from build123d import *

# Parameters (mm, degrees)
SKETCH_W        = 34
SKETCH_H        = 34
PAD_DEPTH       = 80
POCKET_DEPTH    = 80
SKETCH002_R     = 3
POCKET001_DEPTH = 4
SKETCH003_R     = 3
POCKET002_DEPTH = 4
SKETCH004_R     = 4
POCKET003_DEPTH = 2
SKETCH005_R     = 4
POCKET004_DEPTH = 2
SKETCH006_W     = 6.4
SKETCH006_H     = 2
SKETCH006_W_2   = 4
POCKET005_DEPTH = 12
SKETCH007_W     = 6.4
SKETCH007_H     = 2
SKETCH007_W_2   = 4
POCKET006_DEPTH = 12
CHAMFER_SIZE    = 1.98
CHAMFER001_SIZE = 1.98


with BuildPart() as part:
    # Sketch → Pad (new body)
    with BuildSketch(Plane.XY):
        with Locations((17, 17)):
            Rectangle(SKETCH_W, SKETCH_H)
    extrude(amount=PAD_DEPTH)

    # Sketch001 (on Face6 of Pad) → Pocket (cut)
    with BuildSketch(Plane.XY.offset(80)):
        Polygon((6.5, 27.5), (14, 27.5), (14, 23.5), (17, 21), (20, 23.5), (20, 27.5), (27.5, 27.5), (27.5, 19.5), (23.5, 19.5), (21, 17), (23.5, 14), (27.5, 14), (27.5, 6.5), (20, 6.5), (20, 10.5), (17, 13), (14, 10.5), (14, 6.5), (6.5, 6.5), (6.5, 14), (10.5, 14), (13, 17), (10.5, 19.5), (6.5, 19.5), align=None)
    extrude(amount=-POCKET_DEPTH, mode=Mode.SUBTRACT)

    # Sketch002 (on Face2 of Pocket) → Pocket001 (cut)
    with BuildSketch(Plane(origin=(0, 0, 0), x_dir=(0, -1, 0), z_dir=(-1, 0, 0))):
        with Locations((-17, 60)):
            Circle(SKETCH002_R)
        with Locations((-17, 20)):
            Circle(SKETCH002_R)
    extrude(amount=-POCKET001_DEPTH, mode=Mode.SUBTRACT)

    # Sketch003 (on Face3 of Pocket001) → Pocket002 (cut)
    with BuildSketch(Plane.YZ.offset(34)):
        with Locations((17, 60)):
            Circle(SKETCH003_R)
        with Locations((17, 20)):
            Circle(SKETCH003_R)
    extrude(amount=-POCKET002_DEPTH, mode=Mode.SUBTRACT)

    # Sketch004 (on Face1 of Pocket002) → Pocket003 (cut)
    with BuildSketch(Plane(origin=(0, 34, 0), x_dir=(-1, 0, 0), z_dir=(0, 1, 0))):
        with Locations((-27, 60)):
            Circle(SKETCH004_R)
        with Locations((-7, 60)):
            Circle(SKETCH004_R)
        with Locations((-27, 20)):
            Circle(SKETCH004_R)
        with Locations((-7, 20)):
            Circle(SKETCH004_R)
    extrude(amount=-POCKET003_DEPTH, mode=Mode.SUBTRACT)

    # Sketch005 (on Face10 of Pocket003) → Pocket004 (cut)
    with BuildSketch(Plane.XZ):
        with Locations((7, 60)):
            Circle(SKETCH005_R)
        with Locations((27, 60)):
            Circle(SKETCH005_R)
        with Locations((7, 20)):
            Circle(SKETCH005_R)
        with Locations((27, 20)):
            Circle(SKETCH005_R)
    extrude(amount=-POCKET004_DEPTH, mode=Mode.SUBTRACT)

    # Sketch006 (on Face4 of Pocket004) → Pocket005 (cut)
    with BuildSketch(Plane.XY.offset(80)):
        with Locations((17, 1)):
            Rectangle(SKETCH006_W, SKETCH006_H)
        with Locations((17, 7.5)):
            Rectangle(SKETCH006_W_2, SKETCH006_H)
    extrude(amount=-POCKET005_DEPTH, mode=Mode.SUBTRACT)

    # Sketch007 (on Face3 of Pocket005) → Pocket006 (cut)
    with BuildSketch(Plane(origin=(0, 0, 0), x_dir=(1, 0, 0), z_dir=(0, 0, -1))):
        with Locations((17, -1)):
            Rectangle(SKETCH007_W, SKETCH007_H)
        with Locations((17, -7.5)):
            Rectangle(SKETCH007_W_2, SKETCH007_H)
    extrude(amount=-POCKET006_DEPTH, mode=Mode.SUBTRACT)

    # Chamfer
    chamfer_edges = [part.edges().sort_by_distance(p)[0] for p in [
        (17, 2, 12),
    ]]
    chamfer(chamfer_edges, length=CHAMFER_SIZE)

    # Chamfer001
    chamfer001_edges = [part.edges().sort_by_distance(p)[0] for p in [
        (17, 2, 68),
    ]]
    chamfer(chamfer001_edges, length=CHAMFER001_SIZE)


solid = part.part
Input: part model. Units: mm. Frame: model coordinates. A direction names the side the tool comes from. Coordinates: 2 decimals unless noted, no trailing zeros. Loops run counter-clockwise (first coordinate to the right, second up) from the corner with the lowest first, then second, coordinate; pieces in that order, holes last.
Q1. Set-up query: faces 4 (the face through (4, 17, 60)), 5 (the face through (8, 14, 41)), 6 (the face through (17, 8.5, 74)), 7 (the face through (6.479, 0.986, 23.966)). Return all of +Z, -Z, +X, -X, +Y, -Y with unobstructed straight access to the full face (end or side cutting, diameter ignored); none if empty.
Q2. Draft query along X for faces 1 (the face through (30, 17, 60)), 2 (the face through (7, 32, 20)), 3 (the face through (24, 17, 80)). Return one class per face: +X half, -X half, draft (parallel to the pull), parting line (faces both ways), or undercut.
Q3. Cut plane A-A (z = 50). Output: boundary loops of the cut face in (x, y).
Q4. Contact query for flat-ended pins moving along their axis: pin 1 (9 mm diameter, centred on x = 8, z = 60.5, fed in from -Y); pin 2 (3 mm diameter, centred on x = 17, z = 7, fed in from -Y); pin 3 (1.8 mm diameter, centred on y = 18, z = 20, fed in from -X); pin 4 (2 mm diameter, centred on x = 6.5, z = 61, fed in from +Y). Output: stop coordinate, or through.
Q5. Material intervals for line 1 (Z direction, x = 2.35, y = 17); line 2 (Y direction, x = 25.5, z = 39); line 3 (Y direction, x = 11, z = 74.5), sorted ascending.
Q6. Cut plane B-B (z = 73). Give the number of separate pieces and of enclosed holes in the cut face, then the cut area to 3 significant figures.
Working result:
1. face 4: -X
1. face 5: +Z, -Z
1. face 6: +Z
1. face 7: -Y
2. face 1: +X half
2. face 2: undercut
2. face 3: draft
3. outline: (0, 0) - (34, 0) - (34, 34) - (0, 34) - close; hole (6.5, 6.5) - (14, 6.5) - (14, 10.5) - (17, 13) - (20, 10.5) - (20, 6.5) - (27.5, 6.5) - (27.5, 14) - (23.5, 14) - (21, 17) - (23.5, 19.5) - (27.5, 19.5) - (27.5, 27.5) - (20, 27.5) - (20, 23.5) - (17, 21) - (14, 23.5) - (14, 27.5) - (6.5, 27.5) - (6.5, 19.5) - (10.5, 19.5) - (13, 17) - (10.5, 14) - (6.5, 14) - close
4. pin 1: stops at y = 0
4. pin 2: stops at y = 2
4. pin 3: stops at x = 4
4. pin 4: stops at y = 32
5. line 1: z = 0 to 17, 23 to 57, 63 to 80
5. line 2: y = 0 to 6.5, 14 to 19.5, 27.5 to 34
5. line 3: y = 0 to 6.5, 14.6 to 19, 27.5 to 34
6. separate pieces: 1
6. enclosed holes: 2
6. area: 815 mm2
